Answer from the drawing. Dimensions are ordinates in mm from the lowest x, y and z of the part. A direction names the side the tool comes from. Give positions to 0.01 mm unless a question says otherwise; leave off trailing zeros. Write each loop counter-clockwise with the first axis right and the second up, starting at its lowest first coordinate (ties: lowest second). Pieces come first, ordered by that corner, then holes. Notation, with made-up numbers: (2.25, -7) -> (34.25, -7) arc R24 ccw to (34.25, 14) -> close; hole circle Ø3 at (58, 69). An arc over 180 degrees is marked (long way). Write item = value, one per line.
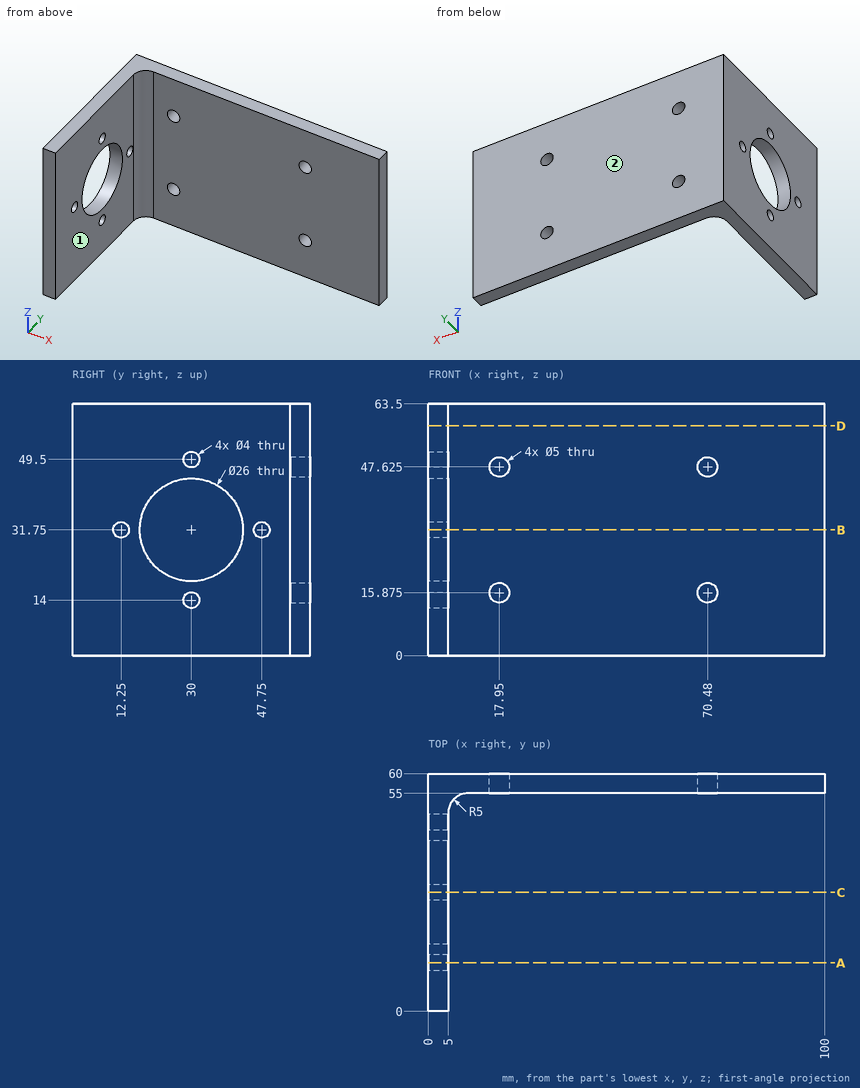
(1) A tool of negligible diameter and unlimited length cuts with its end or side. For the marked faces 1 and 2, from which of +Z, -Z, +X, -X, +Y, -Y can it reach the whole face along a straight path? Write none if from no direction.
Checks:
face_1 = +Z, -Z, +X, -Y
face_2 = +Z, -Z, +X, -X, +Y
(2) The part is cut by section A-A on y = 12.25. Determine the outline of the cut face in (x, z).
Checks:
outline = (0, 0) -> (5, 0) -> (5, 29.75) -> (0, 29.75) -> close; (0, 33.75) -> (5, 33.75) -> (5, 63.5) -> (0, 63.5) -> close
(3) The part is cut by section C-C on y = 30. Determine the outline of the cut face in (x, z).
Checks:
outline = (0, 0) -> (5, 0) -> (5, 12) -> (0, 12) -> close; (0, 16) -> (5, 16) -> (5, 18.75) -> (0, 18.75) -> close; (0, 44.75) -> (5, 44.75) -> (5, 47.5) -> (0, 47.5) -> close; (0, 51.5) -> (5, 51.5) -> (5, 63.5) -> (0, 63.5) -> close
(4) The part is cut by section D-D on z = 58. Determine the outline of the cut face in (x, y), plus the area to 3 significant figures.
Checks:
outline = (0, 0) -> (5, 0) -> (5, 50) arc R5 cw to (10, 55) -> (100, 55) -> (100, 60) -> (0, 60) -> close
area = 780 mm²
(5) Given P1, Ø3.5, axis at y = 30, z = 14, coming from the -X side; P2, Ø3, axis at y = 29, z = 16, coming from the +X side; P3, Ø6.5, axis at x = 17.95, z = 15.88, coming from the -Y side, each flat-ended and moving along its own axis, determine where each tip first touches the part or whether it passes through.
Checks:
P1 = through
P2 = 5
P3 = 55
(6) The part is cut by section B-B on z = 31.75. Determine the outline of the cut face in (x, y).
Checks:
outline = (0, 0) -> (5, 0) -> (5, 10.25) -> (0, 10.25) -> close; (0, 14.25) -> (5, 14.25) -> (5, 17) -> (0, 17) -> close; (0, 43) -> (5, 43) -> (5, 45.75) -> (0, 45.75) -> close; (0, 49.75) -> (5, 49.75) -> (5, 50) arc R5 cw to (10, 55) -> (100, 55) -> (100, 60) -> (0, 60) -> close
(7) Consider L1, parallel to Y at x = 3.2, z = 31.75; L2, parallel to Y at x = 2, z = 14; L3, parallel to Y at x = 52.5, z = 37.5. Determine where each line is inside the solid, lowest interval first.
Checks:
L1 = 0 to 10.25, 14.25 to 17, 43 to 45.75, 49.75 to 60
L2 = 0 to 28, 32 to 60
L3 = 55 to 60
